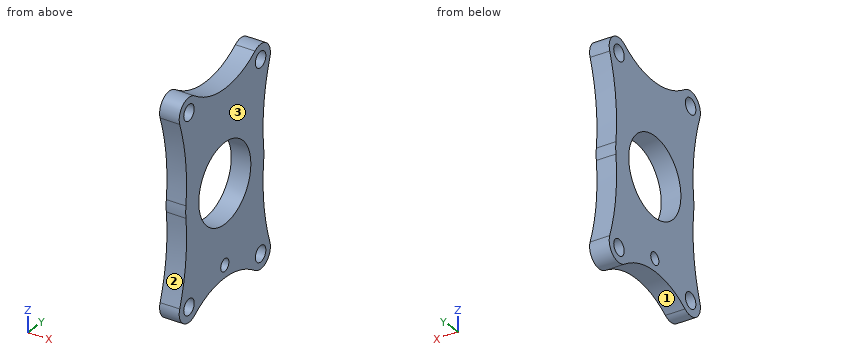
Autodesk Inventor part; units mm, degrees
ref_plane "YZ Plane" through (0, 0, 0) normal (1, 0, 0) x (0, 1, 0)
ref_plane "XZ Plane" through (0, 0, 0) normal (0, 1, 0) x (-1, 0, 0)
ref_plane "XY Plane" through (0, 0, 0) normal (0, 0, 1) x (1, 0, 0)
sketch "Sketch1" plane through (0, 0, 0) normal (1, 0, 0) x (0, 1, 0)
  line L0 (-17.4625, -30.1625) -> (17.4625, -30.1625) construction
  line L1 (17.4625, -30.1625) -> (17.4625, 30.1625) construction
  line L2 (17.4625, 30.1625) -> (-17.4625, 30.1625) construction
  line L3 (-17.4625, 30.1625) -> (-17.4625, -30.1625) construction
  line L4 (-17.4625, -30.1625) -> (17.4625, 30.1625) construction
  line L5 (17.4625, -30.1625) -> (-17.4625, 30.1625) construction
  circle A0 centre (17.4625, 30.1625) radius 4.7625 construction
  circle A1 centre (-17.4625, 30.1625) radius 4.7625 construction
  circle A2 centre (-17.4625, -30.1625) radius 4.7625 construction
  circle A3 centre (17.4625, -30.1625) radius 4.7625 construction
  circle A4 centre (0, 0) radius 12.7
  circle A5 centre (0, 0) radius 19.05 construction
  arc A6 (21.9743, 28.6376) -> (18.9533, 1.9166) centre (82.1311, 8.3053) ccw
  arc A7 (18.9533, -1.9166) -> (21.9743, -28.6376) centre (82.1311, -8.3053) ccw
  arc A8 (14.7053, -34.0457) -> (-14.7053, -34.0457) centre (0, -54.7559) ccw
  arc A9 (-21.9743, -28.6376) -> (-18.9533, -1.9166) centre (-82.1311, -8.3053) ccw
  arc A10 (-18.9533, 1.9166) -> (-21.9743, 28.6376) centre (-82.1311, 8.3053) ccw
  arc A11 (-14.7053, 34.0457) -> (14.7053, 34.0457) centre (0, 54.7559) ccw
  arc A12 (21.9743, 28.6376) -> (14.7053, 34.0457) centre (17.4625, 30.1625) ccw
  arc A13 (14.7053, -34.0457) -> (21.9743, -28.6376) centre (17.4625, -30.1625) ccw
  arc A14 (-21.9743, -28.6376) -> (-14.7053, -34.0457) centre (-17.4625, -30.1625) ccw
  arc A15 (-14.7053, 34.0457) -> (-21.9743, 28.6376) centre (-17.4625, 30.1625) ccw
  arc A16 (-18.9533, 1.9166) -> (-18.9533, -1.9166) centre (0, 0) ccw
  arc A17 (18.9533, -1.9166) -> (18.9533, 1.9166) centre (0, 0) ccw
  point P0 (0, 0)
  point P1 (0, 0)
  point P2 (0, -25.4)
  point P3 (14.7053, -34.0457)
  dimension "d1" = 34.925
  dimension "d2" = 60.325
  dimension "d3" = 25.4
  dimension "d4" = 9.525
  dimension "d5" = 25.4
  dimension "d6" = 6.35
  dimension "d7" = 63.5
  dimension "d8" = 25.4
extrude "Extrusion1" add sketch "Sketch1" along normal blind 6.35
hole "Hole1" at (0, 17.4625, 30.1625) at (0, 17.4625, -30.1625) at (0, -17.4625, -30.1625) at (0, -17.4625, 30.1625) direction (1, 0, 0) diameter 5.1054 end through all
hole "Hole2" at (0, 0, -25.4) direction (1, 0, 0) diameter 3.9624 end through all
properties part number "AR-021" material "Aluminum 6061"
Can you work these out from the model? Positions are in its coordinate system, mm. Face numbers are marked on the shaded views. Round coordinates to 2 decimals unless told otherwise and drop trailing zeros. Order: outer loops, then holes, each group sorted by start corner. A loop starts at its lowest first (then second) coordinate and runs counter-clockwise, first axis right, second up. Notation, with made-up numbers: (33.5, 27.5) -> (57.5, 27.5) arc R28 cw to (57.5, 66.5) -> close; hole circle Ø4 at (66.25, -19.75). An arc over 180 degrees is marked (long way). Return JSON: item names as keys, results as strings. Group by question number.
1. We'd pull the mould along Y, two halves only. Please class the marked faces 1, 2 and 3: released by +Y, released by -Y, zero draft, split by the parting line, or undercut.
2. If we section it at A-A, the plane z = 0: Write out the boundary of the cut face in (x, y), then the cut area to 3 significant figures.
3. Will these pins go through, and if not, where does the flat tip stop? pin 1 (23 mm diameter, centred on y = 0, z = 0, fed in from +X); pin 2 (3 mm diameter, centred on x = 5.5, z = -20.5, fed in from +Y).
4. I need wall thicknesses on line 1 (Z direction, x = 5, y = -17.5); line 2 (Y direction, x = 0.5, z = -28.5); line 3 (Z direction, x = 4, y = 9). Which ranges of each line are inside material? Lowest first, please. Write a range as [from, to].
5. If we section it at D-D, the plane x = 2.5: Write out the boundary of the cut face in (y, z), then the cut area to 3 significant figures.
6. If we section it at B-B, the plane y = 0: Write out the boundary of the cut face in (x, z), then the cut area to 3 significant figures.
7. If we section it at C-C, the plane y = 6.5: Write out the boundary of the cut face in (x, z), then the cut area to 3 significant figures.
Output values:
{
 "1": {"face 1": "undercut", "face 2": "released by -Y", "face 3": "zero draft"},
 "2": {"outline": "(0, -19.05) -> (6.35, -19.05) -> (6.35, -12.7) -> (0, -12.7) -> close; (0, 12.7) -> (6.35, 12.7) -> (6.35, 19.05) -> (0, 19.05) -> close", "area": "80.6 mm²"},
 "3": {"pin 1": "through", "pin 2": "y = 20.13"},
 "4": {"line 1": "[-34.92, -32.71], [-27.61, 27.61], [32.71, 34.92]", "line 2": "[-21.93, -19.4], [-15.53, 15.53], [19.4, 21.93]", "line 3": "[-31, -8.96], [8.96, 31]"},
 "5": {"outline": "(-21.97, -28.64) arc R4.76 ccw to (-14.71, -34.05) arc R25.4 cw to (14.71, -34.05) arc R4.76 ccw to (21.97, -28.64) arc R63.5 cw to (18.95, -1.92) arc R19.05 ccw to (18.95, 1.92) arc R63.5 cw to (21.97, 28.64) arc R4.76 ccw to (14.71, 34.05) arc R25.4 cw to (-14.71, 34.05) arc R4.76 ccw to (-21.97, 28.64) arc R63.5 cw to (-18.95, 1.92) arc R19.05 ccw to (-18.95, -1.92) arc R63.5 cw to start; hole circle Ø5.11 at (-17.46, -30.16); hole circle Ø5.11 at (-17.46, 30.16); hole circle Ø25.4 at (0, 0); hole circle Ø3.96 at (0, -25.4); hole circle Ø5.11 at (17.46, -30.16); hole circle Ø5.11 at (17.46, 30.16)", "area": "1,930 mm²"},
 "6": {"outline": "(0, -29.36) -> (6.35, -29.36) -> (6.35, -27.38) -> (0, -27.38) -> close; (0, -23.42) -> (6.35, -23.42) -> (6.35, -12.7) -> (0, -12.7) -> close; (0, 12.7) -> (6.35, 12.7) -> (6.35, 29.36) -> (0, 29.36) -> close", "area": "186 mm²"},
 "7": {"outline": "(0, -30.2) -> (6.35, -30.2) -> (6.35, -10.91) -> (0, -10.91) -> close; (0, 10.91) -> (6.35, 10.91) -> (6.35, 30.2) -> (0, 30.2) -> close", "area": "245 mm²"}
}
